from build123d import *

# Parameters (mm, degrees)
EXTRUDE_2_DEPTH          = 37.1
SKETCH_2_R               = 1.375
CUT_EXTRUDE_2_DEPTH      = 37.1
CUT_EXTRUDE_3_DEPTH      = 43
CUT_EXTRUDE_3_DEPTH_BACK = 66.1
SKETCH_7_W               = 28.25
SKETCH_7_H               = 55.645233233
CUT_EXTRUDE_4_DEPTH      = 20.1
CUT_EXTRUDE_START        = -51.1
CUT_EXTRUDE_5_DEPTH      = 51.1
SKETCH_11_R              = 1.875
CUT_EXTRUDE_11_DEPTH     = 11
SKETCH_14_R              = 3.8
CUT_EXTRUDE_12_DEPTH     = 2.5
CUT_EXTRUDE_13_DEPTH     = 10
CUT_EXTRUDE_START_2      = -4.5
CUT_EXTRUDE_16_DEPTH     = 4.5
FILLET_1_R               = 3
FILLET_2_R               = 3
FILLET_3_R               = 3
FILLET_4_R               = 3


# Read off the part's stored shape, not the designer's step: 切除-拉伸16
with BuildPart() as part:
    # 草图1 → 凸台-拉伸2 (new body)
    with BuildSketch(Plane.XY):
        with BuildLine():
            Line((-79.849997265, 7.517951971), (-80.824006782, -6.607735752))
            Line((-80.824006782, -6.607735752), (-34.011664697, -9.835590396))
            Line((-34.011664697, -9.835590396), (-33.037718089, 4.289184974))
            ThreePointArc((-33.037718089, 4.289184974), (-31.289416401, 5.37750396), (-29.597256671, 6.551212806))
            ThreePointArc((-29.597256671, 6.551212806), (-28.511524827, 13.53842873), (-35.49874075, 14.624160574))
            ThreePointArc((-35.49874075, 14.624160574), (-56.254713351, 8.628523944), (-75.991651506, 17.415521695))
            ThreePointArc((-75.991651506, 17.415521695), (-83.061756308, 17.298825117), (-82.94505973, 10.228720316))
            ThreePointArc((-82.94505973, 10.228720316), (-81.431142485, 8.834956844), (-79.849997265, 7.517951971))
        make_face()
        with BuildLine():
            ThreePointArc((-35.49874075, 14.624160574), (-28.511524827, 13.53842873), (-29.597256671, 6.551212806))
            ThreePointArc((-29.597256671, 6.551212806), (-19.60326972, 16.966618055), (-13.781348513, 30.175163589))
            ThreePointArc((-13.781348513, 30.175163589), (-17.447406903, 36.221651485), (-23.493894799, 32.555593096))
            ThreePointArc((-23.493894799, 32.555593096), (-27.912943426, 22.529829618), (-35.49874075, 14.624160574))
        make_face()
        with BuildLine():
            ThreePointArc((-95.369360777, 35.795593613), (-91.41450046, 21.915219816), (-82.94505973, 10.228720316))
            ThreePointArc((-82.94505973, 10.228720316), (-83.061756308, 17.298825117), (-75.991651506, 17.415521695))
            ThreePointArc((-75.991651506, 17.415521695), (-82.420263145, 26.28599722), (-85.422145072, 36.821702632))
            ThreePointArc((-85.422145072, 36.821702632), (-90.908807434, 41.282255975), (-95.369360777, 35.795593613))
        make_face()
    extrude(amount=EXTRUDE_2_DEPTH)

    # 草图2 → 切除-拉伸2 (cut)
    with BuildSketch(Plane.XY):
        with Locations((-90.395752924, 36.308648122)):
            Circle(SKETCH_2_R)
        with Locations((-79.468355618, 13.822121005)):
            Circle(SKETCH_2_R)
        with Locations((-56.591693385, 3.749865202)):
            Circle(SKETCH_2_R)
        with Locations((-32.547998711, 10.58768669)):
            Circle(SKETCH_2_R)
        with Locations((-18.637621656, 31.365378342)):
            Circle(SKETCH_2_R)
    extrude(amount=CUT_EXTRUDE_2_DEPTH, mode=Mode.SUBTRACT)

    # 草图7 → 切除-拉伸3 (cut, two sides: drawn at the far end of the back side and taken through both)
    with BuildSketch(Plane(origin=(-33.175735668, 2.287568784, 0), x_dir=(0, 0, -1), z_dir=(0.9976311807721483, -0.0687897314369622, 0)).offset(-CUT_EXTRUDE_3_DEPTH_BACK)):
        with Locations((-18.625, 20.670671677)):
            Rectangle(SKETCH_7_W, SKETCH_7_H)
    extrude(amount=CUT_EXTRUDE_3_DEPTH + CUT_EXTRUDE_3_DEPTH_BACK, mode=Mode.SUBTRACT)

    # 草图8 → 切除-拉伸4 (cut)
    with BuildSketch(Plane(origin=(0, 0, 0), x_dir=(-1, 0, 0), z_dir=(0, 0, -1))):
        with BuildLine():
            ThreePointArc((82.94505973, 10.228720316), (51.234404279, 81.455692616), (29.597256671, 6.551212806))
            ThreePointArc((29.597256671, 6.551212806), (28.511524827, 13.53842873), (35.49874075, 14.624160574))
            ThreePointArc((35.49874075, 14.624160574), (51.922117851, 71.47936814), (75.991651506, 17.415521695))
            ThreePointArc((75.991651506, 17.415521695), (83.061756308, 17.298825117), (82.94505973, 10.228720316))
        make_face()
    extrude(amount=-CUT_EXTRUDE_4_DEPTH, mode=Mode.SUBTRACT)

    # 草图9 → 切除-拉伸5 (cut)
    with BuildSketch(Plane.XY.offset(37.1).offset(CUT_EXTRUDE_START)):
        with BuildLine():
            Line((-80.824006782, -6.607735752), (-76.420204424, -6.911391439))
            Line((-76.420204424, -6.911391439), (-76.076255766, -1.923235535))
            ThreePointArc((-76.076255766, -1.923235535), (-74.504863731, 1.236152849), (-75.627746717, 4.581319764))
            ThreePointArc((-75.627746717, 4.581319764), (-77.78440766, 5.984165292), (-79.849997265, 7.517951971))
            Line((-79.849997265, 7.517951971), (-80.824006782, -6.607735752))
        make_face()
        with BuildLine():
            Line((-38.070187243, -4.543870592), (-38.4141359, -9.532026496))
            Line((-38.4141359, -9.532026496), (-34.011664697, -9.835590396))
            Line((-34.011664697, -9.835590396), (-33.037718089, 4.289184974))
            ThreePointArc((-33.037718089, 4.289184974), (-35.293603575, 3.053877922), (-37.621678194, 1.960684706))
            ThreePointArc((-37.621678194, 1.960684706), (-39.193070229, -1.198703677), (-38.070187243, -4.543870592))
        make_face()
    extrude(amount=CUT_EXTRUDE_5_DEPTH, mode=Mode.SUBTRACT)

    # 草图11 → 切除-拉伸11 (cut)
    with BuildSketch(Plane(origin=(-0.491980372, -7.135003276, 0), x_dir=(0.9976311807721483, -0.06878973143696221, 0), z_dir=(0.06878973143696221, 0.9976311807721483, 0))):
        with Locations(Location((-61.324623812, -14.675100208, 0), (0, 0, 180))):
            Circle(SKETCH_11_R)
        with Locations(Location((-62.811349691, -23.836728616, 0), (0, 0, 180))):
            Circle(SKETCH_11_R)
        with Locations(Location((-50.64108112, -13.419201263, 0), (0, 0, 180))):
            Circle(SKETCH_11_R)
        with Locations(Location((-52.106556415, -22.574899792, 0), (0, 0, 180))):
            Circle(SKETCH_11_R)
    extrude(amount=-CUT_EXTRUDE_11_DEPTH, mode=Mode.SUBTRACT)

    # 草图14 → 切除-拉伸12 (cut)
    with BuildSketch(Plane(origin=(-0.491980372, -7.135003276, 0), x_dir=(0.9976311807721483, -0.06878973143696221, 0), z_dir=(0.06878973143696221, 0.9976311807721483, 0))):
        with Locations(Location((-61.324623812, -14.675100208, 0), (0, 0, 180))):
            Circle(SKETCH_14_R)
        with Locations(Location((-50.64108112, -13.419201263, 0), (0, 0, 180))):
            Circle(SKETCH_14_R)
        with Locations(Location((-52.106556415, -22.574899792, 0), (0, 0, 180))):
            Circle(SKETCH_14_R)
        with Locations(Location((-62.811349691, -23.836728616, 0), (0, 0, 180))):
            Circle(SKETCH_14_R)
    extrude(amount=-CUT_EXTRUDE_12_DEPTH, mode=Mode.SUBTRACT)

    # 草图15 → 切除-拉伸13 (cut)
    with BuildSketch(Plane(origin=(-0.491980372, -7.135003276, 0), x_dir=(0.9976311807721483, -0.06878973143696221, 0), z_dir=(0.06878973143696221, 0.9976311807721483, 0))):
        with BuildLine():
            Line((-75.763746013, -4.5), (-75.763746013, -32.75))
            ThreePointArc((-75.763746013, -32.75), (-69.912979444, -18.625), (-75.763746013, -4.5))
        make_face()
        with BuildLine():
            Line((-37.667434214, -4.5), (-37.667434214, -32.75))
            ThreePointArc((-37.667434214, -32.75), (-43.518200782, -18.625), (-37.667434214, -4.5))
        make_face()
    extrude(amount=-CUT_EXTRUDE_13_DEPTH, mode=Mode.SUBTRACT)

    # 切除-拉伸16 outline → 切除-拉伸16 (cut)
    with BuildSketch(Plane(origin=(0, 0, 0), x_dir=(-1, 0, 0), z_dir=(0, 0, -1)).offset(CUT_EXTRUDE_START_2)):
        with BuildLine():
            ThreePointArc((81.380542879, 11.845750626), (78.607973299, 9.405066939), (75.61824487, 7.235826783))
            ThreePointArc((75.61824487, 7.235826783), (73.942295414, 2.862089757), (75.649513236, -1.499537171))
            ThreePointArc((75.649513236, -1.499537171), (74.493972214, 1.536793977), (75.627746717, 4.581319764))
            ThreePointArc((75.627746717, 4.581319764), (79.444122325, 7.200664067), (82.94505973, 10.228720316))
            ThreePointArc((82.94505973, 10.228720316), (83.061756308, 17.298825118), (75.991651506, 17.415521695))
            ThreePointArc((75.991651506, 17.415521695), (56.254713351, 8.628523944), (35.49874075, 14.624160574))
            ThreePointArc((35.49874075, 14.624160574), (28.511524827, 13.538428729), (29.597256671, 6.551212806))
            ThreePointArc((29.597256671, 6.551212806), (33.481243181, 4.031807781), (37.621678194, 1.960684706))
            ThreePointArc((37.621678194, 1.960684706), (39.193070229, -1.198703678), (38.070187243, -4.543870592))
            ThreePointArc((38.070187243, -4.543870592), (39.703483657, 0.033543341), (37.621678194, 4.425178744))
            ThreePointArc((37.621678194, 4.425178744), (34.175575911, 6.230266238), (30.925090589, 8.367626054))
            ThreePointArc((30.925090589, 8.367626054), (30.255194041, 12.678738279), (34.566306266, 13.348634827))
            ThreePointArc((34.566306266, 13.348634827), (56.363372095, 7.052264676), (77.090290005, 16.280007077))
            ThreePointArc((77.090290005, 16.280007077), (81.452544668, 16.208005289), (81.380542879, 11.845750626))
        make_face()
    extrude(amount=CUT_EXTRUDE_16_DEPTH, mode=Mode.SUBTRACT)

    # 圆角1
    # the kernel refuses this fillet: 3 mm, written as the material it adds along each edge
    with BuildSketch(Plane(origin=(-83.558489622, -1.407312549, 32.75), x_dir=(0, 0, -1), z_dir=(0.9976311807721482, -0.06878973143696218, 0))) as fillet_1_piece_1_section:
        with BuildLine():
            CenterArc((FILLET_1_R, FILLET_1_R), FILLET_1_R, 180, 90)
            Line((0, FILLET_1_R), (0, 0))
            Line((0, 0), (FILLET_1_R, 0))
        make_face()
    fillet_1_piece_1 = extrude(amount=53.096311799, mode=Mode.PRIVATE)
    fillet_1_piece_1 = fillet_1_piece_1 - Plane(origin=(-90.121131909, -0.274826283, 18.625), x_dir=(0.7054317730471289, -0.04864168557507743, 0.707106781186547), z_dir=(0.06878973143696221, 0.9976311807721483, 0)) * Cylinder(19.975766569, 119, mode=Mode.PRIVATE)
    fillet_1_piece_1 = fillet_1_piece_1 - Plane(origin=(-23.931982529, -4.838771253, 18.625), x_dir=(-0.7054317730471323, 0.04864168557507767, 0.7071067811865438), z_dir=(0.06878973143696221, 0.9976311807721483, 0)) * Cylinder(19.975766569, 119, mode=Mode.PRIVATE)
    fillet_1_piece_1 = fillet_1_piece_1 - Plane(origin=(-79.104278891, 1.553296639, 32.082260552), x_dir=(0.6567900874720489, -0.7540734586222076, 0), z_dir=(0, 0, -1)) * Cylinder(4.610336213, 119, mode=Mode.PRIVATE)
    fillet_1_piece_1 = fillet_1_piece_1 - Plane(origin=(-34.593655069, -1.515847467, 32.082260552), x_dir=(-0.6567900874720498, 0.754073458622207, 0), z_dir=(0, 0, -1)) * Cylinder(4.610336213, 119, mode=Mode.PRIVATE)
    add(fillet_1_piece_1)

    # 圆角2
    # the kernel refuses this fillet: 3 mm, written as the material it adds along each edge
    with BuildSketch(Plane(origin=(-83.558489622, -1.407312549, 4.5), x_dir=(0, 0, 1), z_dir=(0.9976311807721482, -0.06878973143696218, 0))) as fillet_2_piece_1_section:
        with BuildLine():
            CenterArc((FILLET_2_R, -FILLET_2_R), FILLET_2_R, 90, 90)
            Line((0, -FILLET_2_R), (0, 0))
            Line((0, 0), (FILLET_2_R, 0))
        make_face()
    fillet_2_piece_1 = extrude(amount=53.096311799, mode=Mode.PRIVATE)
    fillet_2_piece_1 = fillet_2_piece_1 - Plane(origin=(-90.121862606, -0.285423301, 18.625), x_dir=(0.7054317730468341, -0.048641685575091055, 0.7071067811868403), z_dir=(0.06878973143700999, 0.997631180772145, 0)) * Cylinder(19.975766569, 119, mode=Mode.PRIVATE)
    fillet_2_piece_1 = fillet_2_piece_1 - Plane(origin=(-23.932713226, -4.849368272, 18.625), x_dir=(-0.7054317730468341, 0.048641685575091055, 0.7071067811868403), z_dir=(0.06878973143700999, 0.997631180772145, 0)) * Cylinder(19.975766569, 119, mode=Mode.PRIVATE)
    fillet_2_piece_1 = fillet_2_piece_1 - Plane(origin=(-33.361408051, -0.283600448, 5.162419383), x_dir=(-0.74154000103131, -0.670908657620756, 0), z_dir=(0, 0, 1)) * Cylinder(6.35000025, 119, mode=Mode.PRIVATE)
    fillet_2_piece_1 = fillet_2_piece_1 - Plane(origin=(-80.426781476, 2.885301072, 5.162419383), x_dir=(0.7415400009547184, 0.670908657705411, 0), z_dir=(0, 0, 1)) * Cylinder(6.484527605, 119, mode=Mode.PRIVATE)
    fillet_2_piece_1 = fillet_2_piece_1 - Plane(origin=(-79.104278891, 1.553296639, 5.162419383), x_dir=(0.6567900874720489, -0.7540734586222076, 0), z_dir=(0, 0, -1)) * Cylinder(4.610336213, 119, mode=Mode.PRIVATE)
    add(fillet_2_piece_1)

    # 圆角3
    fillet_3_edges = [part.edges().sort_by_distance(p)[0] for p in [
        (-57.417170162, -8.221708967, 37.1),
    ]]
    fillet(fillet_3_edges, radius=FILLET_3_R)

    # 圆角4
    fillet_4_edges = [part.edges().sort_by_distance(p)[0] for p in [
        (-57.417170162, -8.221708967, 0),
    ]]
    fillet(fillet_4_edges, radius=FILLET_4_R)


solid = part.part
Build history of the part. All positions in model axes, mm. A direction names the side the tool comes from. Give positions to 0.01 mm unless a question says otherwise; leave off trailing zeros. Loops run counter-clockwise (first coordinate to the right, second up) from the corner with the lowest first, then second, coordinate; pieces in that order, holes last. Notation, with made-up numbers: (67, -23.5) -> (100, -23.5) arc R27 cw to (100, 13.5) -> close; hole circle Ø1 at (24, -13). An arc over 180 degrees is marked (long way). Answer in a Markdown table with one row per item.
Item 1: Flat gauge pins, fed straight in: P1, Ø2.5, axis at x = -56.59, y = 3.75, coming from the +Z side (3 decimals); P2, Ø10, axis at x = -44.5, z = 31, coming from the -Y side; P3, Ø5, axis at x = -48, z = 7.5, coming from the +Y side. Where does each tip first touch, or does it go through?
Findings below:
| item | result |
|---|---|
| P1 | passes through |
| P2 | stops at y = -9.46 |
| P3 | stops at y = -2.51 |
Item 2: Slice it at B-B on x = -32. Write the cut outline in (y, z), plus the area to 3 significant figures.
Findings below:
| item | result |
|---|---|
| outline | (4.92, 32.75) -> (9.33, 32.75) -> (9.33, 37.1) -> (4.92, 37.1) -> close; (7.61, 0) -> (9.33, 0) -> (9.33, 4.5) -> (7.61, 4.5) -> close; (11.85, 0) -> (13.85, 0) -> (13.85, 4.5) -> (11.85, 4.5) -> close; (11.85, 32.75) -> (17.6, 32.75) -> (17.6, 37.1) -> (11.85, 37.1) -> close |
| area | 60.9 mm² |
Item 3: Probe line 1 along Z through (x, y) = (-79, 16.5); line 2 along Z through (x, y) = (-26.5, 11); line 3 along Z through (x, y) = (-59.5, -5.5). List the from-to ranges inside material, lowest first. Write a range as [from, to].
Findings below:
| item | result |
|---|---|
| line 1 | z = [0, 4.5], [32.75, 37.1] |
| line 2 | z = [32.75, 37.1] |
| line 3 | z = [0.03, 11.68], [17.67, 37.07] |
Item 4: Tool access for faces 1 (the cylindrical face through (-34.223, 6.203, 2.282)), 2 (the cylindrical face through (-31.236, 11.001, 2.218)), 3 (the cylindrical face through (-81.4, 16.26, 2.28)), 4 (the cylindrical face through (-57.28, -2.36, 5.4)), 5 (the flat face through (-76.25, -4.45, 2.22)): list every direction of +Z, -Z, +X, -X, +Y, -Y with a clear straight run to the whole face (end or side of a thin tool).
Findings below:
| item | result |
|---|---|
| face 1 | -Z, +X, -Y |
| face 2 | +Z, -Z |
| face 3 | -Z |
| face 4 | +X, +Y |
| face 5 | +Z, -Z, -X |
Item 5: Mould opens along X. For faces 6 (the flat face through (-38.24, -7, 34.89)), 7 (the cylindrical face through (-57.092, -7.387, 36.198)), 8 (the cylindrical face through (-80.482, 14.751, 34.895)) say: pulls with the +X half, pulls with the -X half, needs draft (parallel to the pull), parting line crosses it, or undercut.
Findings below:
| item | result |
|---|---|
| face 6 | pulls with the +X half |
| face 7 | pulls with the -X half |
| face 8 | undercut |
Item 6: Slice it at C-C on y = 26. Write the cut outline in (x, z).
Findings below:
| item | result |
|---|---|
| outline | (-93.14, 32.75) -> (-82.28, 32.75) -> (-82.28, 37.1) -> (-93.14, 37.1) -> close; (-25.9, 32.75) -> (-15.04, 32.75) -> (-15.04, 37.1) -> (-25.9, 37.1) -> close |
Item 7: Slice it at A-A on y = 20. Write the cut outline in (x, z), plus the area to 3 significant figures.
Findings below:
| item | result |
|---|---|
| outline | (-90.42, 32.75) -> (-78.38, 32.75) -> (-78.38, 37.1) -> (-90.42, 37.1) -> close; (-29.8, 32.75) -> (-17.76, 32.75) -> (-17.76, 37.1) -> (-29.8, 37.1) -> close |
| area | 105 mm² |
